Read the model definition and answer for the solid it produces. Units are mm, in the model's axes. Face numbers are marked on the shaded views. A direction names the side the tool comes from. Give positions to 0.01 mm unless a question says otherwise; leave off trailing zeros. Loops run counter-clockwise (first coordinate to the right, second up) from the corner with the lowest first, then second, coordinate; pieces in that order, holes last.
(1) Find section A-A, the plane x = 78.7. Write down the section's boundary in (y, z).
(2) Find section B-B, the plane y = 186.7. Write down the section's boundary in (x, z).
(3) Find section C-C, the plane z = 25.5. Write down the section's boundary in (x, y), then the cut area to 3 significant figures.
(4) Each of these flat-tipped pins is pushed along its axis until it touches: P1, Ø2, axis at x = 11.3, y = 186.7, coming from the +Z side; P2, Ø0.6, axis at x = 24.5, y = 126.5, coming from the +Z side; P3, Ø1, axis at x = 67, z = 25, coming from the -Y side. Where does it stop, or does it pass through?
(5) Find section D-D, the plane y = 153. Write down the section's boundary in (x, z), then the cut area to 3 significant figures.
(6) Which of the six approach directions +Z, -Z, +X, -X, +Y, -Y give full straight-line access (tool end or side, diameter ignored) to the marked faces 5 and 6?
(7) Determine the mould class of the marked faces 1, 2, 3 and 4 for opening direction Y: pulls with the +Y half, pulls with the -Y half, needs draft (parallel to the pull), parting line crosses it, or undercut.
(8) Straight lines are drawn through the part: probe 1 along Y at (x, z) = (78.7, 18); probe 2 along X at (y, z) = (129.3, 20.5); probe 3 along X at (y, z) = (166, 20). For each, find the intervals that lie inside material, in ascending order.
```python
from build123d import *

# Parameters (mm, degrees)
BOX010_W          = 10
BOX010_H          = 10
BOX010_DEPTH      = 21
FILLET001_R       = 4
ARRAY008_X_COUNT  = 3
ARRAY008_X_PITCH  = 20
BOX008_W          = 70
BOX008_H          = 60
BOX008_DEPTH      = 26
BOX007_W          = 74
BOX007_H          = 64
BOX007_DEPTH      = 26
CYLINDER007_R     = 1.3
CYLINDER007_DEPTH = 26
CYLINDER006_R     = 3.3
CYLINDER006_DEPTH = 26
ARRAY004_X_COUNT  = 2
ARRAY004_X_PITCH  = 67.4
ARRAY004_Y_COUNT  = 2
ARRAY004_Y_PITCH  = 57.4


with BuildPart() as wall_hole_array:
    # Box010 → Box010 (new body)
    with BuildSketch(Plane(origin=(34.5, -4.5, 8), x_dir=(1, 0, 0), z_dir=(0, 0, 1))):
        with Locations((5, 5)):
            Rectangle(BOX010_W, BOX010_H)
    extrude(amount=BOX010_DEPTH)

    # Fillet001
    fillet001_edges = [wall_hole_array.edges().sort_by_distance(p)[0] for p in [
        (34.5, 0.5, 8),
        (44.5, 0.5, 8),
    ]]
    fillet(fillet001_edges, radius=FILLET001_R)

    # Array008 X: wall hole array ×3


with BuildPart() as wall_hole_array_1:
    add(wall_hole_array.part)
    with Locations(*[(i * ARRAY008_X_PITCH, 0, 0) for i in range(1, ARRAY008_X_COUNT)]):
        add(wall_hole_array.part)


with BuildPart() as wall_hole_array_2:
    # Array008 placement: moved
    add(wall_hole_array_1.part.moved(Location((-22.5, 0, 0))))


with BuildPart() as wall_inner_extraction:
    # Box008 → Box008 (new body)
    with BuildSketch(Plane(origin=(2, 2, 0), x_dir=(1, 0, 0), z_dir=(0, 0, 1))):
        with Locations((35, 30)):
            Rectangle(BOX008_W, BOX008_H)
    extrude(amount=BOX008_DEPTH)


with BuildPart() as wall_box_cut:
    # Box007 → Box007 (new body)
    with BuildSketch(Plane.XY):
        with Locations((37, 32)):
            Rectangle(BOX007_W, BOX007_H)
    extrude(amount=BOX007_DEPTH)

    # Cut004: cut wall inner extraction
    add(wall_inner_extraction.part, mode=Mode.SUBTRACT)


with BuildPart() as wall_box_hole:
    # Cylinder007 → Cylinder007 (new body)
    with BuildSketch(Plane.XY):
        Circle(CYLINDER007_R)
    extrude(amount=CYLINDER007_DEPTH)


with BuildPart() as wall_fusion_cut:
    # Cylinder006 → Cylinder006 (new body)
    with BuildSketch(Plane.XY):
        Circle(CYLINDER006_R)
    extrude(amount=CYLINDER006_DEPTH)

    # Cut005: cut wall box hole
    add(wall_box_hole.part, mode=Mode.SUBTRACT)


with BuildPart() as wall_fusion_cut_1:
    # Cut005 placement: moved
    add(wall_fusion_cut.part.moved(Location((3.3, 3.3, 0))))

    # Array004 X: wall fusion cut ×2


with BuildPart() as wall_fusion_cut_2:
    add(wall_fusion_cut_1.part)
    with Locations(*[(i * ARRAY004_X_PITCH, 0, 0) for i in range(1, ARRAY004_X_COUNT)]):
        add(wall_fusion_cut_1.part)

    # Array004 Y: wall fusion cut ×2


with BuildPart() as wall_fusion_cut_3:
    add(wall_fusion_cut_2.part)
    with Locations(*[(0, i * ARRAY004_Y_PITCH, 0) for i in range(1, ARRAY004_Y_COUNT)]):
        add(wall_fusion_cut_2.part)

    # Fusion003: union wall box cut
    add(wall_box_cut.part)


with BuildPart() as wall_fusion_cut_4:
    # Fusion003 placement: moved
    add(wall_fusion_cut_3.part.moved(Location((0, 0, 3))))

    # Cut007: cut wall hole array
    add(wall_hole_array_2.part, mode=Mode.SUBTRACT)


with BuildPart() as wall_fusion_cut_5:
    # Cut007 placement: moved
    add(wall_fusion_cut_4.part.moved(Location((8, 126, 0))))


solid = wall_fusion_cut_5.part
```
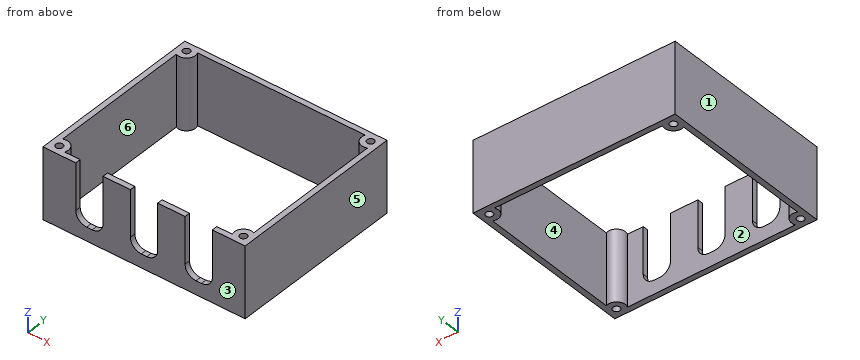
Entries:
1. outline: (126, 3) - (128, 3) - (128, 29) - (126, 29) - close; (130.6, 3) - (132.6, 3) - (132.6, 29) - (130.6, 29) - close; (183.4, 3) - (185.4, 3) - (185.4, 29) - (183.4, 29) - close; (188, 3) - (190, 3) - (190, 29) - (188, 29) - close
2. outline: (8, 3) - (10, 3) - (10, 29) - (8, 29) - close; (12.6, 3) - (14.6, 3) - (14.6, 29) - (12.6, 29) - close; (75.4, 3) - (77.4, 3) - (77.4, 29) - (75.4, 29) - close; (80, 3) - (82, 3) - (82, 29) - (80, 29) - close
3. outline: (8, 126) - (20, 126) - (20, 128) - (14.33, 128) arc R3.3 ccw to (10, 132.33) - (10, 183.67) arc R3.3 ccw to (14.33, 188) - (75.67, 188) arc R3.3 ccw to (80, 183.67) - (80, 132.33) arc R3.3 ccw to (75.67, 128) - (70, 128) - (70, 126) - (82, 126) - (82, 190) - (8, 190) - close; (30, 126) - (40, 126) - (40, 128) - (30, 128) - close; (50, 126) - (60, 126) - (60, 128) - (50, 128) - close; hole circle Ø2.6 at (11.3, 129.3); hole circle Ø2.6 at (11.3, 186.7); hole circle Ø2.6 at (78.7, 129.3); hole circle Ø2.6 at (78.7, 186.7)
3. area: 529 mm2
4. P1: passes through
4. P2: stops at z = 8
4. P3: stops at y = 188
5. outline: (8, 3) - (10, 3) - (10, 29) - (8, 29) - close; (80, 3) - (82, 3) - (82, 29) - (80, 29) - close
5. area: 104 mm2
6. face 5: +Z, -Z, +X, +Y, -Y
6. face 6: +Z, -Z
7. face 1: needs draft
7. face 2: undercut
7. face 3: pulls with the -Y half
7. face 4: undercut
8. probe 1: y = 126 to 128, 130.6 to 132.6, 183.4 to 185.4, 188 to 190
8. probe 2: x = 8 to 10, 12.6 to 14.6, 75.4 to 77.4, 80 to 82
8. probe 3: x = 8 to 10, 80 to 82
